For this review, use the dimensioned drawing (mm, ordinates from the lowest corner) and the shaded views. Round coordinates to 2 decimals unless told otherwise and drop trailing zeros. Loops run counter-clockwise (first coordinate to the right, second up) from the corner with the lowest first, then second, coordinate; pieces in that order, holes last. Notation, with made-up numbers: (57.25, 4) - (86.25, 4) arc R21 cw to (86.25, 29) - close; hole circle Ø11 at (21, -36). An arc over 180 degrees is marked (long way). Return JSON: item names as keys, results as strings. Group by question number.
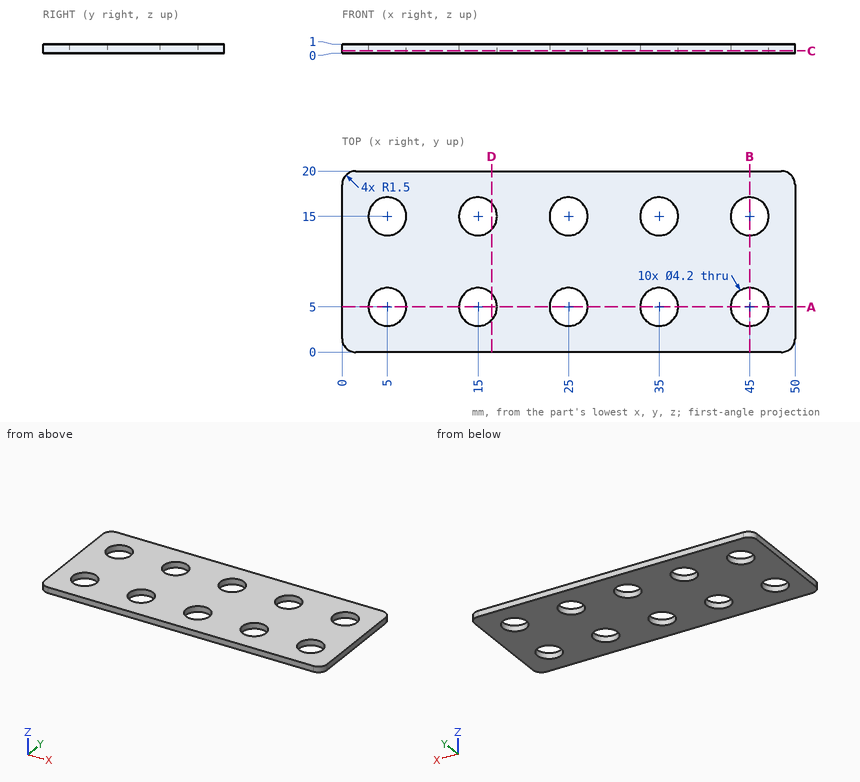
Q1. Add section C-C, the plane z = 0.25. Give the number of separate pieces and of enclosed holes in the cut face, plus the area to 3 significant figures.
Q2. For line 1 (Y direction, x = 15, z = 0.7); line 2 (X direction, y = 16, z = 0.7); line 3 (X direction, y = 4.75, z = 0.1), list the stretches that pass through material, from the lowest coordinate up.
Q3. Add section B-B, the plane x = 45. State the section outline as (y, z) points, plus the area to 3 significant figures.
Q4. Add section A-A, the plane y = 5. State the section outline as (x, z) points.
Q5. Add section D-D, the plane x = 16.5. State the section outline as (y, z) points.
Evaluation:
{
 "1": {"separate pieces": "1", "enclosed holes": "10", "area": "860 mm²"},
 "2": {"line 1": "0 to 2.9, 7.1 to 12.9, 17.1 to 20", "line 2": "0 to 3.15, 6.85 to 13.15, 16.85 to 23.15, 26.85 to 33.15, 36.85 to 43.15, 46.85 to 50", "line 3": "0 to 2.91, 7.09 to 12.91, 17.09 to 22.91, 27.09 to 32.91, 37.09 to 42.91, 47.09 to 50"},
 "3": {"outline": "(0, 0) - (2.9, 0) - (2.9, 1) - (0, 1) - close; (7.1, 0) - (12.9, 0) - (12.9, 1) - (7.1, 1) - close; (17.1, 0) - (20, 0) - (20, 1) - (17.1, 1) - close", "area": "11.6 mm²"},
 "4": {"outline": "(0, 0) - (2.9, 0) - (2.9, 1) - (0, 1) - close; (7.1, 0) - (12.9, 0) - (12.9, 1) - (7.1, 1) - close; (17.1, 0) - (22.9, 0) - (22.9, 1) - (17.1, 1) - close; (27.1, 0) - (32.9, 0) - (32.9, 1) - (27.1, 1) - close; (37.1, 0) - (42.9, 0) - (42.9, 1) - (37.1, 1) - close; (47.1, 0) - (50, 0) - (50, 1) - (47.1, 1) - close"},
 "5": {"outline": "(0, 0) - (3.53, 0) - (3.53, 1) - (0, 1) - close; (6.47, 0) - (13.53, 0) - (13.53, 1) - (6.47, 1) - close; (16.47, 0) - (20, 0) - (20, 1) - (16.47, 1) - close"}
}
